Check sheet for the modelled part. Datum: model origin and axes. Units: mm. A direction names the side the tool comes from. Round coordinates to 2 decimals unless told otherwise and drop trailing zeros. Write each loop counter-clockwise with the first axis right and the second up, starting at its lowest first coordinate (ties: lowest second). Pieces come first, ordered by that corner, then holes. Notation, with made-up numbers: M 81,58 L 85,58 A7 ccw 85,69 Z; hole C 27.25,51 d10. An arc over 180 degrees is marked long. Answer in a Markdown table with one row per item.
```python
from build123d import *

# Parameters (mm, degrees)
F1_DEPTH = 2
F2_R     = 1
F3_DEPTH = 25
F4_R     = 1.020261
F5_DEPTH = 2


with BuildPart() as f1:
    # F0 (on Front) → F1 (new body)
    with BuildSketch(Plane.XZ):
        with BuildLine():
            Line((2.094723, -14.548776), (3, -1.802776))
            ThreePointArc((3, -1.802776), (0, 3.5), (-3, -1.802776))
            Line((-3, -1.802776), (-2.094723, -14.548776))
            ThreePointArc((-2.094723, -14.548776), (0, -16.5), (2.094723, -14.548776))
        make_face()
    extrude(amount=F1_DEPTH)

    # F2 (on face) → F3 (cut)
    with BuildSketch(Plane.XZ.offset(2)):
        Circle(F2_R)
    extrude(amount=-F3_DEPTH, mode=Mode.SUBTRACT)

    # F4 (on face) → F5 (join)
    with BuildSketch(Plane.XZ.offset(2)):
        with Locations((0, -14.4)):
            Circle(F4_R)
    extrude(amount=F5_DEPTH)


solid = f1.part
```
1. Draft check along Z on faces 1 (the face through (0, -1, -1)), 2 (the face through (0, -1, -16.5)), 3 (the face through (0, -2, -6)). Enter one of: +Z half, -Z half, draft (parallel to the pull), parting line (faces both ways), or undercut.
Found:
| item | result |
|---|---|
| face 1 | undercut |
| face 2 | -Z half |
| face 3 | draft |
2. Section check C-C, the plane y = -1.65. Record the cut outline in (x, z).
Found:
| item | result |
|---|---|
| outline | M -3,-1.8 L -2.09,-14.55 A2.1 ccw 2.09,-14.55 L 3,-1.8 A3.5 ccw long Z; hole C 0,0 d2 |
3. Section check A-A, the plane z = 0. Record the cut outline in (x, y).
Found:
| item | result |
|---|---|
| outline | M -3.5,-2 L -1,-2 L -1,0 L -3.5,0 Z; M 1,-2 L 3.5,-2 L 3.5,0 L 1,0 Z |
4. Section check B-B, the plane x = 0. Record the cut outline in (y, z).
Found:
| item | result |
|---|---|
| outline | M -4,-15.42 L -2,-15.42 L -2,-16.5 L 0,-16.5 L 0,-1 L -2,-1 L -2,-13.38 L -4,-13.38 Z; M -2,1 L 0,1 L 0,3.5 L -2,3.5 Z |
5. Section check D-D, the plane y = -3.4. Record the cut outline in (x, z).
Found:
| item | result |
|---|---|
| outline | C 0,-14.4 d2.04 |
6. Go/stop test with flat-tipped pins: pin 1 (2 mm diameter, centred on y = -0.5, z = -8.5, fed in from +X); pin 2 (1.6 mm diameter, centred on x = 0, z = 0, fed in from -Y). Record where each tip stops, or that it passes through.
Found:
| item | result |
|---|---|
| pin 1 | stops at x = 2.6 |
| pin 2 | passes through |
7. Access from +Z, -Z, +X, -X, +Y, -Y to the whole of each face (thin tool, end or side, straight path). Record for faces 4 (the face through (0, 0, -6)), 5 (the face through (-0.2, -3, -15.4)).
Found:
| item | result |
|---|---|
| face 4 | +Z, -Z, +X, -X, +Y |
| face 5 | -Y |
8. Scan lines: L1, parallel to Y at x = 2.25, z = -7.25; L2, parallel to Z at x = -0.75, y = -0.45; L3, parallel to Z at x = -0.25, y = -3.4. Record each from-to range of solid material in increasing order.
Found:
| item | result |
|---|---|
| L1 | y = -2 to 0 |
| L2 | z = -16.36 to -0.66, 0.66 to 3.42 |
| L3 | z = -15.39 to -13.41 |
